Autodesk Fusion 360 part; units mm, degrees
sketch "Esquisse1" plane through (0, 0, 0) normal (0, 0, 1) x (1, 0, 0)
  circle A0 centre (0, 0) radius 22
  circle A1 centre (0, -9) radius 1.7
  circle A2 centre (0, 0) radius 5.5
  circle A3 centre (9, 0) radius 1.7
  circle A4 centre (0, 9) radius 1.7
  circle A5 centre (-9, 0) radius 1.7
  line L0 (0, 0) -> (0, -22) construction
  line L1 (0, 0) -> (0, -20) construction
  line L2 (0, 0) -> (20, 0) construction
  circle A6 centre (0, -19) radius 1.6
  circle A7 centre (16.4545, 9.5) radius 1.6
  circle A8 centre (-16.4545, 9.5) radius 1.6
  point P0 (2.1213, -9.1924)
  point P1 (9.1924, -2.1213)
  point P2 (2.1213, -9.1924)
  point P3 (9.1924, -2.1213)
  point P4 (6.364, -13.435)
  point P5 (13.435, -6.364)
  dimension "d1" = 44
  dimension "d2" = 3.4
  dimension "d3" = 9
  dimension "d4" = 11
  dimension "d6" = 360
  dimension "d17" = 90
  dimension "d18" = 3.2
  dimension "d19" = 19
  dimension "d21" = 360
extrude "Extrusion1" add sketch "Esquisse1" along normal blind 5
The listing builds one solid part. Answer for the finished solid, in the listing's coordinates (mm). Round coordinates to 2 decimals unless told otherwise and drop trailing zeros. Write each loop counter-clockwise with the first axis right and the second up, starting at its lowest first coordinate (ties: lowest second). Pieces come first, ordered by that corner, then holes. Notation, with made-up numbers: M 43.5,40.5 L 53.5,40.5 A22 ccw 53.5,76.5 Z; hole C -4,41 d4. An arc over 180 degrees is marked long. Write each question's results on one line, items separated by ' | '. Start each with the question number.
(1) Each of these flat-tipped pins is pushed along its axis until it touches: P1, Ø2.5, axis at x = -16.45, y = 9.5, coming from the -Z side; P2, Ø1, axis at x = -15, z = 4.5, coming from the +Y side. Where does it stop, or does it pass through?
(2) The part is cut by section D-D, the plane y = 9.5. Write down the section's boundary in (x, z).
(3) Determine the mould class of faces 1 (the flat face through (5, -5, 5)), 2 (the cylindrical face through (-4.769, 21.477, 2.465)), 3 (the cylindrical face through (7.65, 1.03, 2.46)) for opening direction Y: +Y half, -Y half, draft (parallel to the pull), parting line (faces both ways), or undercut.
(4) The part is cut by section A-A, the plane z = 4.2. Give the number of separate pieces and of enclosed holes in the cut face, and give its area (3 significant figures).
(5) Find the intervals of material crossed by line 1 (Y direction, x = 0, z = 3.3); line 2 (Y direction, x = -1, z = 2.5); line 3 (Y direction, x = 2.5, z = 1.15), in increasing order.
(6) The part is cut by section B-B, the plane y = -19. Write down the section's boundary in (x, z), and give its area (3 significant figures).
(7) The part is cut by section C-C, the plane x = 5. Write down the section's boundary in (y, z), and give its area (3 significant figures).
Worked answers:
1) P1: passes through | P2: stops at y = 16.55
2) outline: M -19.84,0 L -18.05,0 L -18.05,5 L -19.84,5 Z; M -14.85,0 L -1.62,0 L -1.62,5 L -14.85,5 Z; M 1.62,0 L 14.85,0 L 14.85,5 L 1.62,5 Z; M 18.05,0 L 19.84,0 L 19.84,5 L 18.05,5 Z
3) face 1: draft | face 2: parting line | face 3: undercut
4) separate pieces: 1 | enclosed holes: 8 | area: 1,370 mm²
5) line 1: y = -22 to -20.6, -17.4 to -10.7, -7.3 to -5.5, 5.5 to 7.3, 10.7 to 22 | line 2: y = -21.98 to -20.25, -17.75 to -10.37, -7.63 to -5.41, 5.41 to 7.63, 10.37 to 21.98 | line 3: y = -21.86 to -4.9, 4.9 to 21.86
6) outline: M -11.09,0 L -1.6,0 L -1.6,5 L -11.09,5 Z; M 1.6,0 L 11.09,0 L 11.09,5 L 1.6,5 Z | area: 94.9 mm²
7) outline: M -21.42,0 L -2.29,0 L -2.29,5 L -21.42,5 Z; M 2.29,0 L 21.42,0 L 21.42,5 L 2.29,5 Z | area: 191 mm²
